```python
from build123d import *

# Parameters (mm, degrees)
SKETCH1_W               = 40
SKETCH1_H               = 40
BOSS_EXTRUDE1_DEPTH     = 40
SKETCH2_W               = 27
SKETCH2_H               = 27
CUT_EXTRUDE1_DEPTH      = 39
SKETCH3_W               = 11
SKETCH3_H               = 6
BOSS_EXTRUDE3_DEPTH     = 6
SKETCH6_W               = 10.5
SKETCH6_H               = 4
CUT_EXTRUDE2_DEPTH      = 4
SKETCH7_W               = 10.5
SKETCH7_H               = 4
CUT_EXTRUDE3_DEPTH      = 4
SKETCH9_R               = 1.5
CUT_EXTRUDE4_DEPTH      = 2
CUT_EXTRUDE5_DEPTH      = 1
CUT_EXTRUDE5_DEPTH_BACK = 2
SKETCH10_R              = 1.5
FILLET3_RADIUS          = 3
FILLET3_LENGTH          = 6
FILLET4_R               = 2
FILLET6_RADIUS          = 3
FILLET6_LENGTH          = 6
FILLET7_R               = 2


with BuildPart() as part:
    # Sketch1 → Boss-Extrude1 (new body)
    with BuildSketch(Plane.XY):
        Rectangle(SKETCH1_W, SKETCH1_H)
    extrude(amount=BOSS_EXTRUDE1_DEPTH)

    # Sketch2 → Cut-Extrude1 (cut)
    with BuildSketch(Plane(origin=(0, 0, 0), x_dir=(-1, 0, 0), z_dir=(0, 0, -1))):
        Rectangle(SKETCH2_W, SKETCH2_H)
    extrude(amount=-CUT_EXTRUDE1_DEPTH, mode=Mode.SUBTRACT)

    # Sketch3 → Boss-Extrude3 (add)
    with BuildSketch(Plane(origin=(0, 0, 0), x_dir=(-1, 0, 0), z_dir=(0, 0, -1))):
        Polygon((-20, 0), (-20, 3), (-31, 3), (-31, 0), (-31, -3), (-20, -3), align=None)
        with Locations((25.5, 0)):
            Rectangle(SKETCH3_W, SKETCH3_H)
    extrude(amount=-BOSS_EXTRUDE3_DEPTH)

    # Sketch6 → Cut-Extrude2 (cut)
    with BuildSketch(Plane(origin=(0, 0, 0), x_dir=(-1, 0, 0), z_dir=(0, 0, -1))):
        with Locations((-18.75, 0.029439605)):
            Rectangle(SKETCH6_W, SKETCH6_H)
    extrude(amount=-CUT_EXTRUDE2_DEPTH, mode=Mode.SUBTRACT)

    # Sketch7 → Cut-Extrude3 (cut)
    with BuildSketch(Plane(origin=(0, 0, 0), x_dir=(-1, 0, 0), z_dir=(0, 0, -1))):
        with Locations((18.75, -0.052667078)):
            Rectangle(SKETCH7_W, SKETCH7_H)
    extrude(amount=-CUT_EXTRUDE3_DEPTH, mode=Mode.SUBTRACT)

    # Sketch9 → Cut-Extrude4 (cut)
    with BuildSketch(Plane(origin=(0, 0, 4), x_dir=(-1, 0, 0), z_dir=(0, 0, -1))):
        with Locations((-18.75, 0.029439605)):
            Circle(SKETCH9_R)
    extrude(amount=-CUT_EXTRUDE4_DEPTH, mode=Mode.SUBTRACT)

    # Sketch10 → Cut-Extrude5 (cut, two sides: drawn at the far end of the back side and taken through both)
    with BuildSketch(Plane(origin=(0, 0, 4), x_dir=(-1, 0, 0), z_dir=(0, 0, -1)).offset(-CUT_EXTRUDE5_DEPTH_BACK)):
        with Locations(Location((18.75, -0.052667078, 0), (0, 0, 33.557309762))):
            Circle(SKETCH10_R)
    extrude(amount=CUT_EXTRUDE5_DEPTH + CUT_EXTRUDE5_DEPTH_BACK, mode=Mode.SUBTRACT)

    # Fillet3: full round fillet: the end face becomes a half cylinder, R = half its width
    fillet3_face = Plane((31, 0, 3), x_dir=(0, 0, -1), z_dir=(1, 0, 0))  # on the end face: x along it, z out of the body
    fillet3_slab = fillet3_face.offset(-FILLET3_RADIUS / 2) * Box(FILLET3_LENGTH, 2 * FILLET3_RADIUS, FILLET3_RADIUS, mode=Mode.PRIVATE)  # the body's end, R deep
    fillet3_round = Plane((28, 0, 3), x_dir=(1, 0, 0), z_dir=(0, 0, -1)) * Cylinder(FILLET3_RADIUS, FILLET3_LENGTH, mode=Mode.PRIVATE)  # its axis R under the face
    add(fillet3_slab - fillet3_round, mode=Mode.SUBTRACT)

    # Fillet4
    fillet4_edges = [part.edges().sort_by_distance(p)[0] for p in [
        (24, -1.970560395, 2),
        (24, 2.029439605, 2),
    ]]
    fillet(fillet4_edges, radius=FILLET4_R - 0.0001)  # a hair under: the kernel refuses the full size

    # Fillet6: full round fillet: the end face becomes a half cylinder, R = half its width
    fillet6_face = Plane((-31, 0, 3), x_dir=(0, 0, -1), z_dir=(-1, 0, 0))  # on the end face: x along it, z out of the body
    fillet6_slab = fillet6_face.offset(-FILLET6_RADIUS / 2) * Box(FILLET6_LENGTH, 2 * FILLET6_RADIUS, FILLET6_RADIUS, mode=Mode.PRIVATE)  # the body's end, R deep
    fillet6_round = Plane((-28, 0, 3), x_dir=(-1, 0, 0), z_dir=(0, 0, -1)) * Cylinder(FILLET6_RADIUS, FILLET6_LENGTH, mode=Mode.PRIVATE)  # its axis R under the face
    add(fillet6_slab - fillet6_round, mode=Mode.SUBTRACT)

    # Fillet7
    fillet7_edges = [part.edges().sort_by_distance(p)[0] for p in [
        (-24, 1.947332922, 2),
        (-24, -2.052667078, 2),
    ]]
    fillet(fillet7_edges, radius=FILLET7_R - 0.0001)  # a hair under: the kernel refuses the full size


solid = part.part
```
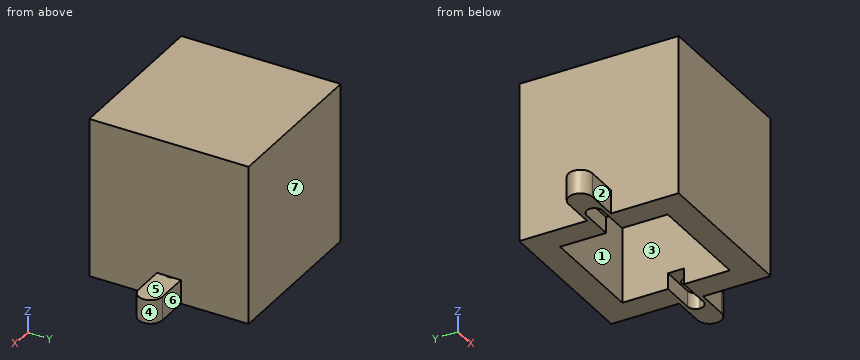
Work out the finished part from the listing and answer in its coordinate system (mm). Face numbers are marked on the shaded views. A direction names the side the tool comes from. Coordinates: 2 decimals unless noted, no trailing zeros. Order: outer loops, then holes, each group sorted by start corner. A loop starts at its lowest first (then second) coordinate and runs counter-clockwise, first axis right, second up. Notation, with made-up numbers: (46, -5) - (53, -5) arc R25 ccw to (53, 17) - close; hole circle Ø10 at (71, 68). An arc over 180 degrees is marked (long way). Answer as a JSON object with one key per item and string values.
1. The mould has two halves that part along X. Classify the marked faces 1, 2, 3 and 4: +X half, -X half, draft (parallel to the pull), parting line (faces both ways), or undercut.
Output values:
{"face 1": "undercut", "face 2": "draft", "face 3": "undercut", "face 4": "+X half"}
2. Find section B-B on x = -7. Determine the outline of the cut face in (y, z), plus the area to 3 significant figures.
Output values:
{"outline": "(-20, 0) - (-13.5, 0) - (-13.5, 39) - (13.5, 39) - (13.5, 0) - (20, 0) - (20, 40) - (-20, 40) - close", "area": "547 mm²"}
3. Find section A-A on z = 24.5. Determine the outline of the cut face in (x, y), plus the area to 3 significant figures.
Output values:
{"outline": "(-20, -20) - (20, -20) - (20, 20) - (-20, 20) - close; hole (-13.5, -13.5) - (13.5, -13.5) - (13.5, 13.5) - (-13.5, 13.5) - close", "area": "871 mm²"}
4. Each of these flat-tipped pins is pushed along its axis until it touches: P1, Ø6, axis at y = 12.5, z = 34, coming from the -X side; P2, Ø2, axis at x = -19.5, y = 1, coming from the -Z side; P3, Ø4, axis at y = 8.5, z = 31, coming from the +X side; P4, Ø13.5, axis at x = 4.5, y = 4, coming from the -Z side. Where does it stop, or does it pass through?
Output values:
{"P1": "stops at x = -20", "P2": "stops at z = 0", "P3": "stops at x = 20", "P4": "stops at z = 39"}
5. A tool of negligible diameter and unlimited length cuts with its end or side. For the marked faces 5, 6 and 7, from which of +Z, -Z, +X, -X, +Y, -Y can it reach the whole face along a straight path? Write none if from no direction.
Output values:
{"face 5": "+Z, +X, +Y, -Y", "face 6": "+Z, -Z, +X, +Y", "face 7": "+Z, -Z, +X, -X, +Y"}
6. Consider line 1 (X direction, y = -4, z = 37); line 2 (Y direction, x = -18.75, z = 4.8). Determine where each line is inside the solid, lowest interval first.
Output values:
{"line 1": "x = -20 to -13.5, 13.5 to 20", "line 2": "y = -20 to -1.55, 1.45 to 20"}
